CAD build for the part. Positions are in the model's coordinates, mm. Face numbers are marked on the shaded views. A direction names the side the tool comes from. Coordinates: 2 decimals unless noted, no trailing zeros. Loops run counter-clockwise (first coordinate to the right, second up) from the corner with the lowest first, then second, coordinate; pieces in that order, holes last.
1) Wall check: line 1 along Y through (x, z) = (8.5, 2.25); line 2 along Y through (x, z) = (6.75, 1.25); line 3 along X through (y, z) = (23.57, 3.1). Give the ranges that are in metal, low to high.
2) Saw through at C-C, the plane y = 23.57. Write the cut outline in (x, z).
3) Saw through at B-B, the plane x = 4.75. Write the cut outline in (y, z), and give its area (3 significant figures).
4) Two-plate mould, pull along Y, no slides. Class the marked faces 3, 4 and 5: +Y half, -Y half, draft (parallel to the pull), parting line (faces both ways), or undercut.
5) Saw through at A-A, the plane x = 8.5. Write the cut outline in (y, z), and give its area (3 significant figures).
6) Saw through at D-D, the plane z = 0.6. Write the cut outline in (x, y).
7) Which spindle directions (+Z, -Z, +X, -X, +Y, -Y) get a long thin tool onto all of the face, cutting with end or side? Do the marked faces 1 and 2. Say none if no direction does.
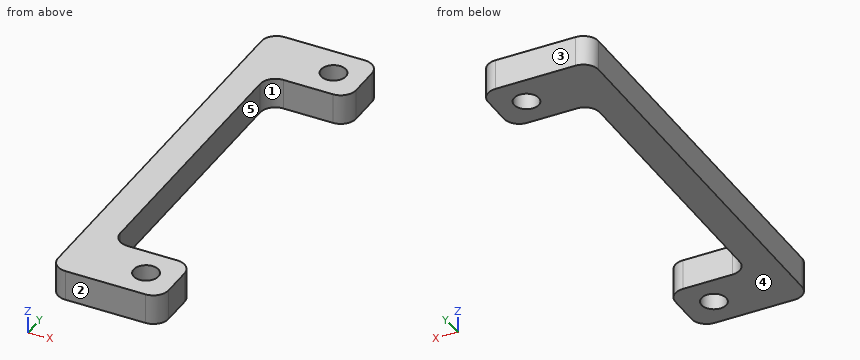
Autodesk Inventor part; units mm, degrees
ref_plane "YZ Plane" through (0, 0, 0) normal (1, 0, 0) x (0, 1, 0)
ref_plane "XZ Plane" through (0, 0, 0) normal (0, 1, 0) x (-1, 0, 0)
ref_plane "XY Plane" through (0, 0, 0) normal (0, 0, 1) x (1, 0, 0)
sketch "Skizze1" plane through (0, 0, 0) normal (0, 0, 1) x (1, 0, 0)
  line L0 (-2, -19.57) -> (2, -19.57)
  line L1 (2, -19.57) -> (2, 19.57)
  line L2 (2, 19.57) -> (-2, 19.57)
  line L3 (-2, 19.57) -> (-2, -19.57)
  line L4 (-2, -19.57) -> (2, 19.57) construction
  line L5 (2, -19.57) -> (-2, 19.57) construction
  line L6 (-2, 19.57) -> (10.5, 19.57)
  line L7 (12.5, 21.57) -> (12.5, 25.57)
  line L8 (10.5, 27.57) -> (0, 27.57)
  line L9 (-2, 25.57) -> (-2, 19.57)
  line L10 (-2, -19.57) -> (10.5, -19.57)
  line L11 (12.5, -21.57) -> (12.5, -25.57)
  line L12 (10.5, -27.57) -> (0, -27.57)
  line L13 (-2, -25.57) -> (-2, -19.57)
  line L14 (8.5, -23.57) -> (8.5, 23.57) construction
  circle A0 centre (8.5, -23.57) radius 4 construction
  circle A1 centre (8.5, 23.57) radius 4 construction
  circle A2 centre (8.5, 23.57) radius 2
  arc A3 (12.5, 25.57) -> (10.5, 27.57) centre (10.5, 25.57) ccw
  arc A4 (10.5, 19.57) -> (12.5, 21.57) centre (10.5, 21.57) ccw
  arc A5 (0, 27.57) -> (-2, 25.57) centre (0, 25.57) ccw
  arc A6 (-2, -25.57) -> (0, -27.57) centre (0, -25.57) ccw
  arc A7 (10.5, -27.57) -> (12.5, -25.57) centre (10.5, -25.57) ccw
  arc A8 (12.5, -21.57) -> (10.5, -19.57) centre (10.5, -21.57) ccw
  point P0 (0, 0)
  point P1 (12.5, -27.57)
  dimension "d0" = 47.14
  dimension "d1" = 6.5
  dimension "d2" = 4
  dimension "d3" = 8
  dimension "d4" = 4
  dimension "d5" = 2
extrude "Extrusion1" add sketch "Skizze1" along normal blind 4 contours L3 L2 L1 L0 | L0 L10 A8 L11 A7 L12 A6 L13 | L9 A5 L8 A3 L7 A4 L6 L2 | A2
hole "Bohrung1" at (8.5, 23.57, 0) at (8.5, -23.57, 0) direction (0, 0, 1) diameter 3.242 depth 11.8 tip angle 118
fillet "Rundung1" radius 2 2 edges at (2, -19.57, 2) (2, 19.57, 2)
properties part number "Nema23_24Mount" material "Aluminium 6061"
Data:
1. line 1: y = -27.57 to -25.19, -21.95 to -19.57, 19.57 to 21.95, 25.19 to 27.57
1. line 2: y = -27.57 to -19.57, 19.57 to 27.57
1. line 3: x = -2 to 6.88, 10.12 to 12.5
2. outline: (-2, 0) - (6.88, 0) - (6.88, 4) - (-2, 4) - close; (10.12, 0) - (12.5, 0) - (12.5, 4) - (10.12, 4) - close
3. outline: (-27.57, 0) - (-19.57, 0) - (-19.57, 4) - (-27.57, 4) - close; (19.57, 0) - (27.57, 0) - (27.57, 4) - (19.57, 4) - close
3. area: 64.0 mm2
4. face 3: +Y half
4. face 4: draft
4. face 5: undercut
5. outline: (-27.57, 0) - (-25.19, 0) - (-25.19, 4) - (-27.57, 4) - close; (-21.95, 0) - (-19.57, 0) - (-19.57, 4) - (-21.95, 4) - close; (19.57, 0) - (21.95, 0) - (21.95, 4) - (19.57, 4) - close; (25.19, 0) - (27.57, 0) - (27.57, 4) - (25.19, 4) - close
5. area: 38.1 mm2
6. outline: (-2, -25.57) arc R2 ccw to (0, -27.57) - (10.5, -27.57) arc R2 ccw to (12.5, -25.57) - (12.5, -21.57) arc R2 ccw to (10.5, -19.57) - (4, -19.57) arc R2 cw to (2, -17.57) - (2, 17.57) arc R2 cw to (4, 19.57) - (10.5, 19.57) arc R2 ccw to (12.5, 21.57) - (12.5, 25.57) arc R2 ccw to (10.5, 27.57) - (0, 27.57) arc R2 ccw to (-2, 25.57) - close; hole circle Ø3.24 at (8.5, -23.57); hole circle Ø3.24 at (8.5, 23.57)
7. face 1: +Z, -Z, +X
7. face 2: +Z, -Z, +X, -X, -Y
